Here's how the part is built. I have some questions about the finished solid (model axes, mm). A direction names the side the tool comes from. Round coordinates to 2 decimals unless told otherwise and drop trailing zeros. Order: outer loops, then holes, each group sorted by start corner. A loop starts at its lowest first (then second) coordinate and runs counter-clockwise, first axis right, second up.
Autodesk Inventor part; units mm, degrees
ref_plane "Work Plane1" through (-50.9068, 28.5, 21.3) normal (0, 0, 1) x (1, 0, 0)
ref_plane "YZ Plane" through (0, 0, 0) normal (1, 0, 0) x (0, 1, 0)
ref_plane "XZ Plane" through (0, 0, 0) normal (0, 1, 0) x (-1, 0, 0)
sketch "Sketch1" plane through (0, 0, 0) normal (0, 0, 1) x (1, 0, 0)
  line L0 (0, -12.35) -> (-250, -12.35)
  line L1 (0, -12.35) -> (0, -7.2)
  line L2 (0, -7.2) -> (-250, -7.2)
  line L3 (-250, -12.35) -> (-250, -7.2)
  line L4 (-250, 5.15) -> (0, 5.15)
  line L5 (-250, 0) -> (-250, 5.15)
  line L6 (0, 0) -> (-250, 0)
  line L7 (0, 0) -> (0, 5.15)
  line L8 (0, 6.4) -> (-250, 6.4)
  line L9 (-250, -13.6) -> (0, -13.6)
  line L10 (-159.051, -15.85) -> (90.949, -15.85)
  line L11 (-159.051, -21) -> (-159.051, -15.85)
  line L12 (90.949, -21) -> (-159.051, -21)
  line L13 (90.949, -21) -> (90.949, -15.85)
  line L14 (90.949, 8.65) -> (-159.051, 8.65)
  line L15 (90.949, 13.8) -> (90.949, 8.65)
  line L16 (-159.051, 13.8) -> (90.949, 13.8)
  line L17 (-159.051, 13.8) -> (-159.051, 8.65)
  line L18 (-159.051, 7.4) -> (90.949, 7.4)
  line L19 (90.949, -14.6) -> (-159.051, -14.6)
  line L20 (-159.051, -34.6) -> (90.949, -34.6)
  line L21 (90.949, 27.4) -> (-159.051, 27.4)
  line L22 (-50.9068, -42.05) -> (-6.1068, -42.05)
  line L23 (-6.1068, -42.05) -> (-6.1068, -35.7)
  line L24 (-50.9068, -35.7) -> (-6.1068, -35.7)
  line L25 (-50.9068, -42.05) -> (-50.9068, -35.7)
  line L26 (-50.9068, 28.5) -> (-6.1068, 28.5)
  line L27 (-6.1068, 28.5) -> (-6.1068, 34.85)
  line L28 (-50.9068, 34.85) -> (-6.1068, 34.85)
  line L29 (-50.9068, 28.5) -> (-50.9068, 34.85)
  line L30 (-50.9068, -42.05) -> (-50.9068, 34.85) construction
  line L31 (-6.1068, -42.05) -> (-6.1068, 34.85) construction
  line L32 (-50.9068, -13.6) -> (-6.1068, -13.6)
  line L33 (-6.1068, 6.4) -> (-50.9068, 6.4)
  line L34 (-50.9068, 6.4) -> (-50.9068, -13.6)
  line L35 (-6.1068, -13.6) -> (6.5932, -13.6)
  line L36 (6.5932, -13.6) -> (6.5932, 6.4)
  line L37 (6.5932, 6.4) -> (-6.1068, 6.4)
  line L38 (-28.5068, -35.7) -> (-28.5068, 28.5) construction
  line L39 (6.5932, -13.6) -> (-6.1068, 6.4) construction
  circle A0 centre (0.2432, -3.6) radius 2.75
  circle A1 centre (-28.5068, -3.6) radius 2.75
  line L40 (6.5932, 6.4) -> (-50.9068, 6.4)
  line L41 (-50.9068, 6.4) -> (-50.9068, -13.6)
  line L42 (-50.9068, -13.6) -> (6.5932, -13.6)
  line L43 (6.5932, -13.6) -> (6.5932, 6.4)
  dimension "d0" = 12.7
  dimension "d1" = 5.5
extrude "Extrusion1" add sketch "Sketch1" along normal blind 6.35 contours L1 L2 L34 L6 L7 L4 L8 L37 L36 L35 L9 L0 | L0 L34 L2 L1 | L34 L4 L7 L6
sketch "Sketch2" plane through (0, 0, 6.35) normal (0, 0, 1) x (1, 0, 0)
  line L0 (-50.9068, -13.6) -> (6.5932, -13.6)
  line L1 (6.5932, -13.6) -> (6.5932, 6.4)
  line L2 (-50.9068, -13.6) -> (6.5932, -13.6)
  line L3 (6.5932, -13.6) -> (6.5932, -9.79)
  line L4 (6.5932, -9.79) -> (-50.9068, -9.79)
  line L5 (-50.9068, -9.79) -> (-50.9068, -13.6)
  line L6 (6.5932, 6.4) -> (-50.9068, 6.4)
  line L7 (-50.9068, 6.4) -> (6.5932, 6.4)
  line L8 (6.5932, 6.4) -> (6.5932, 2.59)
  line L9 (6.5932, 2.59) -> (-50.9068, 2.59)
  line L10 (-50.9068, 2.59) -> (-50.9068, 6.4)
  point P0 (0, 0)
  dimension "d4" = 3.81
ref_plane "Work Plane1" through (-50.9068, 28.5, 21.3) normal (0, 0, 1) x (1, 0, 0)
extrude "Extrusion2" add sketch "Sketch2" along normal up to surface (14.95 mm away)
sketch "Sketch3" plane through (6.5932, -13.6, 0) normal (1, 0, 0) x (0, 0, -1)
  line L0 (-21.3, 16.19) -> (-21.3, 20)
  line L1 (0, 0) -> (-21.3, 0)
  line L2 (-21.3, 0) -> (-21.3, 20)
  line L3 (-21.3, 20) -> (0, 20)
  line L4 (0, 20) -> (0, 0)
  point P0 (0, 13.6)
extrude "Extrusion3" add sketch "Sketch3" along normal blind 6.35
sketch "Sketch5" plane through (-50.9068, -13.6, 0) normal (-1, 0, 0) x (0, 0, 1)
  line L0 (21.3, 0) -> (0, 0)
  line L1 (21.3, 20) -> (21.3, 0)
  line L2 (0, 0) -> (21.3, 0)
  line L3 (21.3, 0) -> (21.3, 20)
  line L4 (21.3, 20) -> (0, 20)
  line L5 (0, 20) -> (0, 0)
  point P0 (0, 13.6)
extrude "Extrusion4" add sketch "Sketch5" against normal blind 3.81
sketch "Sketch6" plane through (-50.9068, -13.6, 0) normal (0, -1, 0) x (1, 0, 0)
  circle A0 centre (9.9, 11.4) radius 2.5
  circle A1 centre (34.9, 11.4) radius 2.5
  point P0 (50.9068, 0)
extrude "Extrusion5" cut sketch "Sketch6" against normal through all
sketch "Sketch7" plane through (-50.9068, -13.6, 0) normal (0, -1, 0) x (1, 0, 0)
  circle A0 centre (9.9, 11.4) radius 2.5
  circle A1 centre (34.9, 11.4) radius 2.5
  line L0 (0, 0) -> (63.85, 0)
  line L1 (63.85, 21.3) -> (63.85, 0)
  line L2 (0, 21.3) -> (63.85, 21.3)
  line L3 (0, 0) -> (0, 21.3)
  point P0 (50.9068, 0)
extrude "Extrusion6" add sketch "Sketch7" along normal blind 0.9
sketch "Sketch8" plane through (-50.9068, 6.4, 21.3) normal (0, 1, 0) x (1, 0, 0)
  circle A0 centre (9.9, 9.9) radius 2.5
  circle A1 centre (34.9, 9.9) radius 2.5
  line L0 (0, 0) -> (63.85, 0)
  line L1 (63.85, 21.3) -> (63.85, 0)
  line L2 (0, 21.3) -> (63.85, 21.3)
  line L3 (0, 21.3) -> (0, 0)
  point P0 (50.9068, 21.3)
extrude "Extrusion7" add sketch "Sketch8" along normal blind 0.9
sketch "Sketch9" plane through (-50.9068, 7.3, 21.3) normal (0, 1, 0) x (1, 0, 0)
  point P0 (50.9068, 21.3)
properties part number "rollerHolderInnerZ"
1. If we section it at A-A, the plane z = 11.4: Write out the boundary of the cut face in (x, y).
Evaluation:
outline: (-50.91, -14.5) - (-43.51, -14.5) - (-43.51, -9.79) - (-47.1, -9.79) - (-47.1, 2.59) - (-43.51, 2.59) - (-43.51, 7.3) - (-50.91, 7.3) - close; (-38.51, -14.5) - (-18.51, -14.5) - (-18.51, -9.79) - (-38.51, -9.79) - close; (-38.51, 2.59) - (-18.51, 2.59) - (-18.51, 7.3) - (-38.51, 7.3) - close; (-13.51, -14.5) - (12.94, -14.5) - (12.94, 7.3) - (-13.51, 7.3) - (-13.51, 2.59) - (6.59, 2.59) - (6.59, -9.79) - (-13.51, -9.79) - close
2. If we section it at B-B, the plane y = 3.25: Write out the boundary of the cut face in (x, z), and give its area (3 significant figures).
Evaluation:
outline: (-50.91, 0) - (12.94, 0) - (12.94, 21.3) - (-50.91, 21.3) - close; hole circle Ø5 at (-41.01, 11.4); hole circle Ø5 at (-16.01, 11.4)
area: 1,320 mm2
3. On a 3-axis mill with a long thin cutter (end or side, diameter ignored), from which of +Z, -Z, +X, -X, +Y, -Y can I reach the whole of each face in a straight line? I mean faces 1 (the flat face through (-19, 7.3, 11)), 2 (the flat face through (-20, -9.79, 14)). Say none if no direction works.
Evaluation:
face 1: +Z, -Z, +X, -X, +Y
face 2: +Z
4. I'm going to push flat-ended pins straight in: P1, Ø5, axis at x = -28.51, y = -3.6, coming from the -Z side; P2, Ø8, axis at x = -31.5, y = -3, coming from the +Z side. Where does each tip first touch, or does it pass through?
Evaluation:
P1: passes through
P2: stops at z = 6.35
5. If we section it at D-D, the plane z = 1.75: Write out the boundary of the cut face in (x, y).
Evaluation:
outline: (-50.91, -14.5) - (12.94, -14.5) - (12.94, 7.3) - (-50.91, 7.3) - close; hole circle Ø5.5 at (-28.51, -3.6); hole circle Ø5.5 at (0.24, -3.6)
6. I need wall thicknesses on probe 1 along X at (y, z) = (5.3, 11.4); probe 2 along Y at (x, z) = (-9.5, 20.75); probe 3 along X at (y, z) = (1.5, 18). Which ranges of each line are inside material? Lowest first, please.
Evaluation:
probe 1: x = -50.91 to -43.51, -38.51 to -18.51, -13.51 to 12.94
probe 2: y = -14.5 to -9.79, 2.59 to 7.3
probe 3: x = -50.91 to -47.1, 6.59 to 12.94
7. If we mould it in two halves opening along Z, with no side actions, what happens to faces 3 (the flat face through (-19, -4, 0)), 4 (the cylindrical face through (-13.62, 4.91, 12.15)), 5 (the flat face through (-21, -4, 6.35)), 6 (the flat face through (-50.907, -4, 11))? For each: released by +Z, released by -Z, zero draft, split by the parting line, or undercut.
Evaluation:
face 3: released by -Z
face 4: undercut
face 5: released by +Z
face 6: zero draft
8. If we section it at C-C, the plane x = -45.5: Write out the boundary of the cut face in (y, z).
Evaluation:
outline: (-14.5, 0) - (7.3, 0) - (7.3, 21.3) - (2.59, 21.3) - (2.59, 6.35) - (-9.79, 6.35) - (-9.79, 21.3) - (-14.5, 21.3) - close
